Verification items for the finished model (mm, model axes). A direction names the side the tool comes from. Round coordinates to 2 decimals unless told otherwise and drop trailing zeros. Loops run counter-clockwise (first coordinate to the right, second up) from the corner with the lowest first, then second, coordinate; pieces in that order, holes last.
from build123d import *

# Parameters (mm, degrees)
F0_W     = 127
F0_H     = 127
F1_DEPTH = 25.4
F2_W     = 25.4
F2_H     = 127
F3_DEPTH = 101.6
F4_W     = 101.6
F4_H     = 25.4
F5_DEPTH = 101.6
F6_W     = 25.4
F6_H     = 25.4
F7_DEPTH = 25.4


with BuildPart() as f1:
    # F0 (on Top) → F1 (new body)
    with BuildSketch(Plane.XY):
        with Locations((7.114284, -3.634389)):
            Rectangle(F0_W, F0_H)
    extrude(amount=F1_DEPTH)

    # F2 (on face) → F3 (join)
    with BuildSketch(Plane.XY.offset(25.4)):
        with Locations((-43.685716, -3.634389)):
            Rectangle(F2_W, F2_H)
    extrude(amount=F3_DEPTH)

    # F4 (on face) → F5 (join)
    with BuildSketch(Plane.XY.offset(25.4)):
        with Locations((19.814284, 47.165611)):
            Rectangle(F4_W, F4_H)
    extrude(amount=F5_DEPTH)

    # F6 (on face) → F7 (cut)
    with BuildSketch(Plane.XY.offset(25.4)):
        with Locations((57.914284, -54.434389)):
            Rectangle(F6_W, F6_H)
    extrude(amount=-F7_DEPTH, mode=Mode.SUBTRACT)


solid = f1.part
1. Section check A-A (z = 27.5). Enter the section's corners in (x, y).
2. Tool access check on faces 1 (the face through (6, -3, 0)), 2 (the face through (58, -41.734, 13)), 3 (the face through (19, 34.466, 75)). Record the directions out of +Z, -Z, +X, -X, +Y, -Y that give a thin tool (end or side, any length) a straight path to the whole face; none if there is none.
3. Scan lines: L1, parallel to Y at x = 39.5, z = 73.5; L2, parallel to X at y = 2, z = 70; L3, parallel to Z at x = 44, y = 3. Record each from-to range of solid material in increasing order.
4. Gauge pin test, flat ends, axial feed: P1, Ø5, axis at y = -3, z = 92, coming from the +X side; P2, Ø12.5, axis at x = 54.5, z = 16, coming from the -Y side; P3, Ø1.5, axis at x = 41.5, y = 31, coming from the +Z side. Record the tip position at first contact, or that the pin passes through.
5. Section check B-B (y = -57). Enter the section's corners in (x, z).
Taken from the geometry:
1. outline: (-56.39, -67.13) - (-30.99, -67.13) - (-30.99, 34.47) - (70.61, 34.47) - (70.61, 59.87) - (-56.39, 59.87) - close
2. face 1: -Z, +X, -X, +Y, -Y
2. face 2: +Z, -Z, +X, -Y
2. face 3: +Z, +X, -Y
3. L1: y = 34.47 to 59.87
3. L2: x = -56.39 to -30.99
3. L3: z = 0 to 25.4
4. P1: stops at x = -30.99
4. P2: stops at y = -41.73
4. P3: stops at z = 25.4
5. outline: (-56.39, 0) - (45.21, 0) - (45.21, 25.4) - (-30.99, 25.4) - (-30.99, 127) - (-56.39, 127) - close
